from build123d import *

# Parameters (mm, degrees)
F0_W     = 19.05
F0_H     = 6.35
F1_DEPTH = 25.4
F2_DEPTH = 12.7
F4_DEPTH = 25.4


with BuildPart() as f1:
    # F0 (on Top) → F1 (new body)
    with BuildSketch(Plane.XY):
        Polygon((19.05, 25.4), (0, 25.4), (0, 19.05), (8.733842, 19.05), (8.733842, 6.35), (0, 6.35), (0, 0), (19.05, 0), align=None)
        with Locations((-9.525, 3.175)):
            Rectangle(F0_W, F0_H)
        with Locations((-9.525, 22.225)):
            Rectangle(F0_W, F0_H)
    extrude(amount=F1_DEPTH)

    # F0 (on Top) → F2 (join)
    with BuildSketch(Plane.XY):
        Polygon((0, 19.05), (-19.05, 19.05), (-19.05, 6.35), (0, 6.35), (8.733842, 6.35), (8.733842, 19.05), align=None)
    extrude(amount=F2_DEPTH)

    # F3 (on face) → F4 (cut)
    with BuildSketch(Plane.XZ):
        Polygon((19.05, 25.4), (0, 25.4), (19.05, 0), align=None)
    extrude(amount=-F4_DEPTH, mode=Mode.SUBTRACT)


solid = f1.part
Design review of the part built by this model. Coordinates are the model's own, in mm. A direction names the side the tool comes from. Give positions to 0.01 mm unless a question says otherwise; leave off trailing zeros. Loops run counter-clockwise (first coordinate to the right, second up) from the corner with the lowest first, then second, coordinate; pieces in that order, holes last. Notation, with made-up numbers: (19.25, 81.25) - (67.25, 81.25) arc R21 ccw to (67.25, 103.25) - close; hole circle Ø9 at (50.5, 77). An arc over 180 degrees is marked (long way). Write item = value, one per line.
1) Draft analysis for pull direction Y (two halves, no side actions). For faces 1 (the face through (11.508, 12.522, 10.056)), 2 (the face through (8.734, 13, 13)), 3 (the face through (-8, 19.05, 19)), 4 (the face through (-4, 25.4, 13)), state which applies: +Y half, -Y half, draft (parallel to the pull), parting line (faces both ways), or undercut.
Result sheet:
face_1 = draft
face_2 = undercut
face_3 = undercut
face_4 = +Y half
2) Take a section at D-D on z = 5. State the section outline as (x, y) points, and give its area (3 significant figures).
Result sheet:
outline = (-19.05, 0) - (15.3, 0) - (15.3, 25.4) - (-19.05, 25.4) - close
area = 872 mm2
3) Tool access review of faces 5 (the face through (-10, 22, 25.4)), 6 (the face through (-5, 13, 12.7)): name each direction out of +Z, -Z, +X, -X, +Y, -Y from which nothing blocks a thin tool from reaching the whole face with its end or side.
Result sheet:
face_5 = +Z, +X, -X, +Y, -Y
face_6 = +Z, -X
4) Take a section at A-A on z = 16. State the section outline as (x, y) points, and give its area (3 significant figures).
Result sheet:
outline = (-19.05, 0) - (7.05, 0) - (7.05, 6.35) - (-19.05, 6.35) - close; (-19.05, 19.05) - (7.05, 19.05) - (7.05, 25.4) - (-19.05, 25.4) - close
area = 331 mm2
5) Take a section at C-C on y = 8.5. State the section outline as (x, z) points.
Result sheet:
outline = (-19.05, 0) - (19.05, 0) - (8.73, 13.75) - (8.73, 12.7) - (-19.05, 12.7) - close
6) Clearance check with flat-ended pins moving along their axes: pin 1 Ø3 at (y, z) = (20.5, 9) entering from +X (3 decimals); pin 2 Ø0.5 at (y, z) = (12.5, 13.5) entering from -X; pin 3 Ø4 at (y, z) = (9, 11) entering from +X. State where each tip first meets the part, or that it passes through.
Result sheet:
pin_1 = 13.425
pin_2 = 8.73
pin_3 = 12.3
7) To check wall thickness, follow line 1 (Y direction, x = -11, z = 20.25); line 2 (Z direction, x = 7, y = 7.5); line 3 (X direction, y = 7.5, z = 2.5) (3 decimals). State the ranges of each line that lie inside material, in increasing order.
Result sheet:
line_1 = 0 to 6.35, 19.05 to 25.4
line_2 = 0 to 12.7
line_3 = -19.05 to 17.175
8) Take a section at B-B on x = -4. State the section outline as (y, z) points, and give its area (3 significant figures).
Result sheet:
outline = (0, 0) - (25.4, 0) - (25.4, 25.4) - (19.05, 25.4) - (19.05, 12.7) - (6.35, 12.7) - (6.35, 25.4) - (0, 25.4) - close
area = 484 mm2
